Source: CAD feature listing. Evaluate the final solid. Frame: model axes, mm. A direction names the side the tool comes from. Give positions to 0.01 mm unless a question says otherwise; leave off trailing zeros. Order: outer loops, then holes, each group sorted by start corner. A loop starts at its lowest first (then second) coordinate and runs counter-clockwise, first axis right, second up. Notation, with made-up numbers: M 69,74.5 L 95,74.5 A18 ccw 95,81.5 Z; hole C 71.25,18.5 d1. An arc over 180 degrees is marked long. Use CSV: the item, a comma, the result in double quotes. Start each with the question number.
Item 1: Section query C-C on x = -49. Return loops of the section in (y, z).
Item 2: Section query D-D on z = 32. Return loops of the section in (x, y).
Item 3: Ray query, probe 1 along Z at (x, y) = (-14.5, 0.5); probe 2 along Y at (x, z) = (44.5, 3.75); probe 3 along Z at (x, y) = (39, -3.75). Return the intervals inside material, ascending. Write a range as from..to.
Item 4: Access query for faces 5 (the face through (56.14, -3.57, 3.22)), 6 (the face through (1, -1, 37.695)), 7 (the face through (42.19, -0.96, 3.13)), 8 (the face through (-48, 0, 6.35)), 9 (the face through (9.505, 3.4, 37.6)). Directions: +Z, -Z, +X, -X, +Y, -Y. A direction counts if a zero-diameter tool reaches every point of the face in a straight line with its end or side. Return the directions, or none.
Item 5: First-contact query: pin 1 (6 mm diameter, centred on y = 0, z = 45.5, fed in from +X); pin 2 (4 mm diameter, centred on y = 1.5, z = 59.5, fed in from -X); pin 3 (2 mm diameter, centred on y = -0.5, z = 58, fed in from +X); pin 4 (3 mm diameter, centred on x = -44.5, y = 0, fed in from +Z). Flat tips, straight axial feed; report the tip coordinate or a pass-through.
Item 6: Section query B-B on z = 11.35. Return loops of the section in (x, y), and give its area (3 significant figures).
Item 7: Section query A-A on x = 44.5. Return loops of the section in (y, z), and give its area (4 significant figures).
Item 8: Pull-direction query (X, two-part tool) for faces 1 (the face through (-13.5, 0.1, 11.3)), 2 (the face through (0.24, -0.07, 66.35)), 3 (the face through (25.716, -0.07, 31.657)), 4 (the face through (47.4, 0.1, 6.35)); classes: +X half, -X half, draft (parallel to the pull), parting line (faces both ways), or undercut.
from build123d import *

# Parameters (mm, degrees)
SKETCH1_W              = 115.000000124
SKETCH1_H              = 10
BOSS_EXTRUDE1_DEPTH    = 6.35
BOSS_EXTRUDE3_DEPTH    = 10
M2_5_CLEARANCE_HOLE1_D = 3.1
SKETCH8_W              = 18.22
SKETCH8_H              = 11.68
CUT_EXTRUDE3_DEPTH     = 1.75
SKETCH8_9_W            = 18.22
SKETCH8_9_H            = 4.5
CUT_EXTRUDE4_DEPTH     = 89.366127601
FILLET2_R              = 4.7625
F_5_0MM_DOWEL_HOLE1_D  = 5
CUT_EXTRUDE5_DEPTH     = 89.366127601


with BuildPart() as part:
    # Sketch1 → Boss-Extrude1 (new body)
    with BuildSketch(Plane.XY):
        Rectangle(SKETCH1_W, SKETCH1_H)
    extrude(amount=BOSS_EXTRUDE1_DEPTH)

    # Sketch2 → Boss-Extrude3 (add)
    with BuildSketch(Plane.XZ.offset(5)):
        with BuildLine():
            Line((-37.500000062, 6.35), (37.500000062, 6.35))
            Line((37.500000062, 6.35), (13.598116374, 57.681763663))
            ThreePointArc((13.598116374, 57.681763663), (0, 66.35), (-13.598116374, 57.681763663))
            Line((-13.598116374, 57.681763663), (-37.500000062, 6.35))
        make_face()
    extrude(amount=-BOSS_EXTRUDE3_DEPTH)

    # M2.5 Clearance Hole1 (through all)
    with Locations(Plane(origin=(0, 5, 0), x_dir=(1, 0, 0), z_dir=(0, 1, 0))):
        with Locations((6.005, -45.875)):
            Hole(M2_5_CLEARANCE_HOLE1_D / 2)

    # Sketch8 → Cut-Extrude3 (cut)
    with BuildSketch(Plane(origin=(0, 5, 0), x_dir=(-1, 0, 0), z_dir=(0, 1, 0))):
        with Locations((-0.395, 43.535)):
            Rectangle(SKETCH8_W, SKETCH8_H)
    extrude(amount=-CUT_EXTRUDE3_DEPTH, mode=Mode.SUBTRACT)

    # Sketch8<9> → Cut-Extrude4 (cut, through all)
    with BuildSketch(Plane(origin=(0, 5, 0), x_dir=(-1, 0, 0), z_dir=(0, 1, 0))):
        with Locations((-0.395, 35.445)):
            Rectangle(SKETCH8_9_W, SKETCH8_9_H)
    extrude(amount=-CUT_EXTRUDE4_DEPTH, mode=Mode.SUBTRACT)

    # Fillet2
    fillet2_edges = [part.edges().sort_by_distance(p)[0] for p in [
        (-57.500000062, -5, 3.175),
        (-57.500000062, 5, 3.175),
        (57.500000062, 5, 3.175),
        (57.500000062, -5, 3.175),
    ]]
    fillet(fillet2_edges, radius=FILLET2_R)

    # Ø5.0mm Dowel Hole1 (through all)
    with Locations(Plane.XY.offset(6.35)):
        with Locations((44.5, 0), (-44.5, 0)):
            Hole(F_5_0MM_DOWEL_HOLE1_D / 2)

    # Sketch11 → Cut-Extrude5 (cut, through all)
    with BuildSketch(Plane(origin=(0, 5, 0), x_dir=(1, 0, 0), z_dir=(0, 1, 0))):
        with BuildLine():
            Line((-20.000000062, -9.85), (-15.000000062, -9.85))
            ThreePointArc((-15.000000062, -9.85), (-13.500000062, -11.35), (-15.000000062, -12.85))
            Line((-15.000000062, -12.85), (-20.000000062, -12.85))
            ThreePointArc((-20.000000062, -12.85), (-21.500000062, -11.35), (-20.000000062, -9.85))
        make_face()
        with BuildLine():
            Line((-20.000000062, -19.85), (-15.000000062, -19.85))
            ThreePointArc((-15.000000062, -19.85), (-13.500000062, -21.35), (-15.000000062, -22.85))
            Line((-15.000000062, -22.85), (-20.000000062, -22.85))
            ThreePointArc((-20.000000062, -22.85), (-21.500000062, -21.35), (-20.000000062, -19.85))
        make_face()
    extrude(amount=-CUT_EXTRUDE5_DEPTH, mode=Mode.SUBTRACT)


solid = part.part
Verdict:
1,outline,"M -5,0 L 5,0 L 5,6.35 L -5,6.35 Z"
2,outline,"M -25.56,-5 L 25.56,-5 L 25.56,5 L -25.56,5 Z"
3,probe 1,"0..9.94, 12.76..19.94, 22.76..55.74"
3,probe 2,"-5..-2.5, 2.5..5"
3,probe 3,"0..6.35"
4,face 5,"+Z, -Z, +X, -Y"
4,face 6,"+Y, -Y"
4,face 7,"+Z, -Z"
4,face 8,"+Z, -X, +Y, -Y"
4,face 9,"+Y"
5,pin 1,"x = 20.67"
5,pin 2,"x = -13.68"
5,pin 3,"x = 13.92"
5,pin 4,"through"
6,outline,"M -35.17,-5 L -21.5,-5 L -21.5,5 L -35.17,5 Z; M -13.5,-5 L 35.17,-5 L 35.17,5 L -13.5,5 Z"
6,area,"623 mm2"
7,outline,"M -5,0 L -2.5,0 L -2.5,6.35 L -5,6.35 Z; M 2.5,0 L 5,0 L 5,6.35 L 2.5,6.35 Z"
7,area,"31.75 mm2"
8,face 1,"undercut"
8,face 2,"parting line"
8,face 3,"+X half"
8,face 4,"draft"
